The listing builds one solid part. Answer for the finished solid, in the listing's coordinates (mm). A direction names the side the tool comes from. Give positions to 0.01 mm unless a question says otherwise; leave off trailing zeros. Loops run counter-clockwise (first coordinate to the right, second up) from the corner with the lowest first, then second, coordinate; pieces in that order, holes last. Notation, with made-up numbers: (71, 59) - (119, 59) arc R22 cw to (119, 77) - close; hole circle Ø2 at (-26, 14). An arc over 180 degrees is marked (long way). Write each question's results on one line, items separated by ' | '.
from build123d import *

# Parameters (mm, degrees)
SKETCH_1_R      = 1.35
EXTRUDE_1_DEPTH = 3


with BuildPart() as part:
    # 草图1 → 凸台-拉伸1 (new body)
    with BuildSketch(Plane(origin=(0, 0, 0), x_dir=(-1, 0, 0), z_dir=(0, 0, -1))):
        with BuildLine():
            Line((15.657318156, 3), (15.657318156, 20.9998))
            ThreePointArc((15.657318156, 20.9998), (14.7786385, 23.121120344), (12.657318156, 23.9998))
            Line((12.657318156, 23.9998), (-13.843681844, 23.9998))
            Line((-13.843681844, 23.9998), (-24.001092054, 23.467804703))
            ThreePointArc((-24.001092054, 23.467804703), (-26.020271299, 22.537010177), (-26.844181844, 20.471910982))
            Line((-26.844181844, 20.471910982), (-26.844181844, 3.528889024))
            ThreePointArc((-26.844181844, 3.528889024), (-26.020372671, 1.463896655), (-24.001386189, 0.533010723))
            Line((-24.001386189, 0.533010723), (-13.843681844, 0))
            Line((-13.843681844, 0), (12.657318156, 0))
            ThreePointArc((12.657318156, 0), (14.7786385, 0.878679656), (15.657318156, 3))
        make_face()
        with Locations(Location((-24.044031844, 3.501148349, 0), (0, 0, 180))):
            Circle(SKETCH_1_R, mode=Mode.SUBTRACT)
        with Locations(Location((-24.044031844, 20.498351651, 0), (0, 0, 180))):
            Circle(SKETCH_1_R, mode=Mode.SUBTRACT)
        with Locations(Location((3.156018156, 20.498351651, 0), (0, 0, 180))):
            Circle(SKETCH_1_R, mode=Mode.SUBTRACT)
        with Locations(Location((3.156018156, 3.501148349, 0), (0, 0, 180))):
            Circle(SKETCH_1_R, mode=Mode.SUBTRACT)
        with Locations(Location((12.657468156, 2.95, 0), (0, 0, 180))):
            Circle(SKETCH_1_R, mode=Mode.SUBTRACT)
        with Locations(Location((12.657468156, 21.049, 0), (0, 0, 180))):
            Circle(SKETCH_1_R, mode=Mode.SUBTRACT)
        Polygon((-4.343381844, 20.9998), (-4.343381844, 17.9998), (1.156518156, 17.9998), (1.156518156, 6), (-4.343381844, 6), (-4.343381844, 3), (-16.343381844, 3), (-16.343381844, 6), (-21.843181844, 6), (-21.843181844, 17.9998), (-16.343381844, 17.9998), (-16.343381844, 20.9998), align=None, mode=Mode.SUBTRACT)
    extrude(amount=-EXTRUDE_1_DEPTH)


solid = part.part
Item 1: Find the intervals of material crossed by line 1 along X through (y, z) = (14.75, 2.6); line 2 along Y through (x, z) = (-3, 1.05); line 3 along X through (y, z) = (2.95, 0.8), in increasing order. Write a range as [from, to].
Values found:
line 1: x = [-15.66, -1.16], [21.84, 26.84] | line 2: y = [0, 2.16], [4.84, 19.16], [21.84, 24] | line 3: x = [-15.66, -14.01], [-11.31, -4.39], [-1.92, 22.81], [25.28, 26.79]
Item 2: A cutting plane is placed at B-B, the plane x = 10.5. Determine the outline of the cut face in (y, z), plus the area to 3 significant figures.
Values found:
outline: (0, 0) - (3, 0) - (3, 3) - (0, 3) - close; (21, 0) - (24, 0) - (24, 3) - (21, 3) - close | area: 18.0 mm²
Item 3: For faces 5 (the face through (4.343, 5, 1)), 6 (the face through (-4, 12, 3)), determine the directions among +Z, -Z, +X, -X, +Y, -Y from which every point of the face is accessible in a straight line to the end or side of a thin tool.
Values found:
face 5: +Z, -Z | face 6: +Z, +X, -X, +Y, -Y
Item 4: For a pull along X with two mould halves and no side action, classify faces 1 (the face through (1, 0, 1)), 2 (the face through (16.343, 4, 1)), 3 (the face through (-15.657, 12, 1)), 4 (the face through (26.844, 12, 1)) as released by +X, released by -X, zero draft, split by the parting line, or undercut.
Values found:
face 1: zero draft | face 2: undercut | face 3: released by -X | face 4: released by +X
Item 5: A cutting plane is placed at A-A, the plane y = 11.75. Determine the outline of the cut face in (x, z).
Values found:
outline: (-15.66, 0) - (-1.16, 0) - (-1.16, 3) - (-15.66, 3) - close; (21.84, 0) - (26.84, 0) - (26.84, 3) - (21.84, 3) - close
Item 6: A cutting plane is placed at C-C, the plane z = 1.4. Determine the outline of the cut face in (x, y), plus the area to 3 significant figures.
Values found:
outline: (-15.66, 3) arc R3 ccw to (-12.66, 0) - (13.84, 0) - (24, 0.53) arc R3 ccw to (26.84, 3.53) - (26.84, 20.47) arc R3 ccw to (24, 23.47) - (13.84, 24) - (-12.66, 24) arc R3 ccw to (-15.66, 21) - close; hole circle Ø2.7 at (-12.66, 2.95); hole circle Ø2.7 at (-12.66, 21.05); hole circle Ø2.7 at (-3.16, 3.5); hole circle Ø2.7 at (-3.16, 20.5); hole (-1.16, 6) - (4.34, 6) - (4.34, 3) - (16.34, 3) - (16.34, 6) - (21.84, 6) - (21.84, 18) - (16.34, 18) - (16.34, 21) - (4.34, 21) - (4.34, 18) - (-1.16, 18) - close; hole circle Ø2.7 at (24.04, 3.5); hole circle Ø2.7 at (24.04, 20.5) | area: 622 mm²
Item 7: A flat-ended cylindrical pin translates along its axis: P1, Ø0.9, axis at x = 20, z = 2, coming from the +Y side. Find the tip coordinate at first contact, or state that the pin passes through.
Values found:
P1: stops at y = 23.7
Item 8: A cutting plane is placed at D-D, the plane x = 24.5. Determine the outline of the cut face in (y, z).
Values found:
outline: (0.6, 0) - (2.23, 0) - (2.23, 3) - (0.6, 3) - close; (4.77, 0) - (19.23, 0) - (19.23, 3) - (4.77, 3) - close; (21.77, 0) - (23.4, 0) - (23.4, 3) - (21.77, 3) - close
